```python
from build123d import *

# Parameters (mm, degrees)
F0_R     = 9.92251
F1_DEPTH = 44.45
F2_R     = 10.3251
F3_DEPTH = 7.9375
F4_W     = 73.025
F4_H     = 76.2
F5_DEPTH = 57.151
F6_R     = 6.35
F7_R     = 4.7625
F8_R     = 12.7


with BuildPart() as f1:
    # F0 (on Right) → F1 (new body, symmetric)
    with BuildSketch(Plane.YZ):
        with BuildLine():
            Line((0, 44.45), (0, 0))
            Line((0, 0), (57.15, 0))
            Line((57.15, 0), (57.15, 44.45))
            ThreePointArc((57.15, 44.45), (48.7805762724, 64.6555762724), (28.575, 73.025))
            ThreePointArc((28.575, 73.025), (8.3694237276, 64.6555762724), (0, 44.45))
        make_face()
        with Locations((28.575, 44.45)):
            Circle(F0_R, mode=Mode.SUBTRACT)
    extrude(amount=F1_DEPTH, both=True)

    # F2 (on Top) → F3 (join)
    with BuildSketch(Plane.XY):
        with BuildLine():
            Line((22.225, 57.15), (-22.225, 57.15))
            Line((-22.225, 57.15), (-22.225, -53.975))
            ThreePointArc((-22.225, -53.975), (-15.7154482119, -69.6904482119), (0, -76.2))
            ThreePointArc((0, -76.2), (15.7154482119, -69.6904482119), (22.225, -53.975))
            Line((22.225, -53.975), (22.225, 57.15))
        make_face()
        with Locations((0, -53.975)):
            Circle(F2_R, mode=Mode.SUBTRACT)
        with Locations((0, -15.875)):
            Circle(F2_R, mode=Mode.SUBTRACT)
    extrude(amount=F3_DEPTH)

    # F4 (on Front) → F5 (cut, through all)
    with BuildSketch(Plane.XZ):
        with Locations((0, 46.0375)):
            Rectangle(F4_W, F4_H)
    extrude(amount=-F5_DEPTH, mode=Mode.SUBTRACT)

    # F6
    f6_edges = [f1.edges().sort_by_distance(p)[0] for p in [
        (-22.225, 0, 3.96875),
        (22.225, 0, 3.96875),
    ]]
    fillet(f6_edges, radius=F6_R)

    # F7
    f7_edges = [f1.edges().sort_by_distance(p)[0] for p in [
        (-36.5125, 28.575, 7.9375),
        (36.5125, 28.575, 7.9375),
    ]]
    fillet(f7_edges, radius=F7_R)

    # F8
    f8_edges = [f1.edges().sort_by_distance(p)[0] for p in [
        (-44.45, 28.575, 0),
        (44.45, 28.575, 0),
    ]]
    fillet(f8_edges, radius=F8_R)


solid = f1.part
```
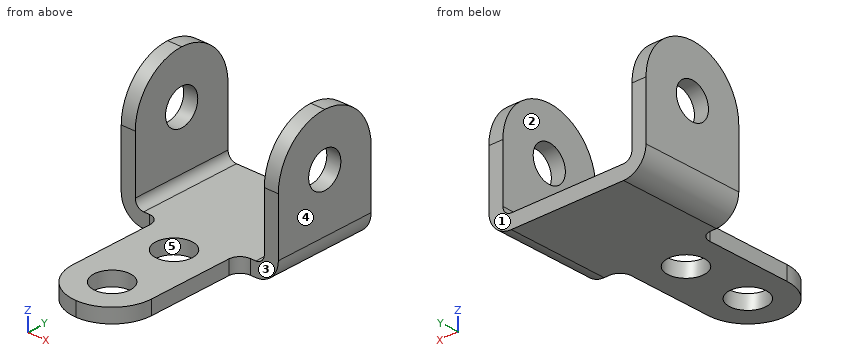
Read the model definition and answer for the solid it produces. Units are mm, in the model's axes. Face numbers are marked on the shaded views. A direction names the side the tool comes from. Give positions to 0.01 mm unless a question says otherwise; leave off trailing zeros. Order: outer loops, then holes, each group sorted by start corner. A loop starts at its lowest first (then second) coordinate and runs counter-clockwise, first axis right, second up. Notation, with made-up numbers: (-12, 66.5) -> (-8, 66.5) arc R24 ccw to (-8, 88.5) -> close; hole circle Ø2 at (79, -15.5). An arc over 180 degrees is marked (long way). One line per item, written item: value. Start each with the question number.
(1) Straight lines are drawn through the part: L1, parallel to Y at x = 0, z = 2; L2, parallel to X at y = 22, z = 21.5; L3, parallel to Y at x = -42, z = 44. For each, find the intervals that lie inside material, in ascending order.
(2) The part is cut by section B-B (y = 22.5). State how many separate pieces and enclosed holes the cut face has, and give its area (3 significant figures).
(3) The part is cut by section C-C (y = -9.5). Determine the outline of the cut face in (x, z) (1 decimal), and give its area (3 significant figures).
(4) The part is cut by section D-D (y = -37.5). Determine the outline of the cut face in (x, z) (1 decimal), and give its area (3 significant figures).
(5) The part is cut by section A-A (z = 29). Determine the outline of the cut face in (x, y).
(6) Flat-ended cylindrical pins translate along their axes: P1, Ø5, axis at x = -37.5, z = 11.5, coming from the -Y side; P2, Ø1, axis at x = -12, y = -60.5, coming from the +Z side; P3, Ø6.5, axis at y = -41.5, z = 6, coming from the -X side (3 decimals). Find the tip coordinate at first contact, or state that the pin passes through.
(7) A tool of negligible diameter and unlimited length cuts with its end or side. For the marked faces 1 and 2, from which of +Z, -Z, +X, -X, +Y, -Y can it reach the whole face along a straight path? Write none if from no direction.
(8) For a pull along Y with two mould halves and no side action, classify the marked faces 3, 4 and 5 as released by +Y, released by -Y, zero draft, split by the parting line, or undercut.
Taken from the geometry:
1. L1: -76.2 to -64.3, -43.65 to -26.2, -5.55 to 57.15
1. L2: -44.45 to -36.51, 36.51 to 44.45
1. L3: 0 to 18.66, 38.49 to 57.15
2. separate pieces: 3
2. enclosed holes: 0
2. area: 1,420 mm^2
3. outline: (-22.2, 0) -> (-8.1, 0) -> (-8.1, 7.9) -> (-22.2, 7.9) -> close; (8.1, 0) -> (22.2, 0) -> (22.2, 7.9) -> (8.1, 7.9) -> close
3. area: 224 mm^2
4. outline: (-22.2, 0) -> (22.2, 0) -> (22.2, 7.9) -> (-22.2, 7.9) -> close
4. area: 353 mm^2
5. outline: (-44.45, 0) -> (-36.51, 0) -> (-36.51, 57.15) -> (-44.45, 57.15) -> close; (36.51, 0) -> (44.45, 0) -> (44.45, 57.15) -> (36.51, 57.15) -> close
6. P1: y = 0
6. P2: z = 7.94
6. P3: x = -22.225
7. face 1: +Z, -Z, +X, -X, +Y
7. face 2: +Z, +Y, -Y
8. face 3: released by -Y
8. face 4: zero draft
8. face 5: undercut
